Model file for the job. Use its own axes, mm. Face numbers are marked on the shaded views. A direction names the side the tool comes from. Coordinates: 2 decimals unless noted, no trailing zeros. Order: outer loops, then holes, each group sorted by start corner. A loop starts at its lowest first (then second) coordinate and runs counter-clockwise, first axis right, second up. Notation, with made-up numbers: M -7,73 L 4,73 A18 cw 4,104 Z; hole C 5,72.5 d11. An arc over 180 degrees is marked long. Return JSON: item names as keys, results as strings.
```python
from build123d import *

# Parameters (mm, degrees)
SKETCH_1_W      = 1800
SKETCH_1_H      = 870
EXTRUDE_1_DEPTH = 70
SKETCH_2_W      = 100
SKETCH_2_H      = 300
EXTRUDE_2_DEPTH = 150
SKETCH_3_W      = 300
SKETCH_3_H      = 300
EXTRUDE_3_DEPTH = 190
SKETCH_4_W      = 90
SKETCH_4_H      = 710
SKETCH_4_W_2    = 1460
SKETCH_4_H_2    = 90
EXTRUDE_4_DEPTH = 70
SKETCH_5_W      = 90
SKETCH_5_H      = 90
EXTRUDE_5_DEPTH = 600
EXTRUDE_6_REACH = 2071.251
SKETCH_6_W      = 90
SKETCH_6_H      = 90
EXTRUDE_7_REACH = 2013.641
SKETCH_7_W      = 650
SKETCH_7_H      = 90


with BuildPart() as part:
    # ｽｹｯﾁ1 → ﾎﾞｽ - 押し出し1 (new body)
    with BuildSketch(Plane(origin=(0, 0, 0), x_dir=(1, 0, 0), z_dir=(0, 1, 0))):
        with Locations((900, 435)):
            Rectangle(SKETCH_1_W, SKETCH_1_H)
    extrude(amount=EXTRUDE_1_DEPTH)

    # ｽｹｯﾁ2 → ﾎﾞｽ - 押し出し2 (add)
    with BuildSketch(Plane(origin=(0, 70, 0), x_dir=(1, 0, 0), z_dir=(0, 1, 0))):
        with Locations((350, 50)):
            Rectangle(SKETCH_2_W, SKETCH_2_H)
        with Locations((1450, 50)):
            Rectangle(SKETCH_2_W, SKETCH_2_H)
        with Locations((1450, 820)):
            Rectangle(SKETCH_2_W, SKETCH_2_H)
        with Locations((350, 820)):
            Rectangle(SKETCH_2_W, SKETCH_2_H)
    extrude(amount=EXTRUDE_2_DEPTH)

    # ｽｹｯﾁ3 → ﾎﾞｽ - 押し出し3 (add)
    with BuildSketch(Plane(origin=(0, 70, 0), x_dir=(1, 0, 0), z_dir=(0, 1, 0))):
        with Locations((900, 435)):
            Rectangle(SKETCH_3_W, SKETCH_3_H)
    extrude(amount=EXTRUDE_3_DEPTH)

    # ｽｹｯﾁ4 → ﾎﾞｽ - 押し出し4 (add)
    with BuildSketch(Plane(origin=(0, 0, 0), x_dir=(-1, 0, 0), z_dir=(0, -1, 0))):
        with Locations((-1675, 435)):
            Rectangle(SKETCH_4_W, SKETCH_4_H)
        with Locations((-900, 715)):
            Rectangle(SKETCH_4_W_2, SKETCH_4_H_2)
        with Locations((-900, 155)):
            Rectangle(SKETCH_4_W_2, SKETCH_4_H_2)
        with Locations((-125, 435)):
            Rectangle(SKETCH_4_W, SKETCH_4_H)
    extrude(amount=EXTRUDE_4_DEPTH)

    # ｽｹｯﾁ5 → ﾎﾞｽ - 押し出し5 (add)
    with BuildSketch(Plane(origin=(0, -70, 0), x_dir=(-1, 0, 0), z_dir=(0, -1, 0))):
        with Locations((-1675, 155)):
            Rectangle(SKETCH_5_W, SKETCH_5_H)
        with Locations((-1675, 715)):
            Rectangle(SKETCH_5_W, SKETCH_5_H)
        with Locations((-125, 155)):
            Rectangle(SKETCH_5_W, SKETCH_5_H)
        with Locations((-125, 715)):
            Rectangle(SKETCH_5_W, SKETCH_5_H)
    extrude(amount=EXTRUDE_5_DEPTH)

    # ｽｹｯﾁ6 → ﾎﾞｽ - 押し出し6 (add, up to next)
    with BuildSketch(Plane(origin=(0, 0, -200), x_dir=(-1, 0, 0), z_dir=(0, 0, -1)), mode=Mode.PRIVATE) as extrude_6_sk1:
        with Locations((-1675, -525)):
            Rectangle(SKETCH_6_W, SKETCH_6_H)
    extrude_6_tool1 = extrude(extrude_6_sk1.sketch, amount=EXTRUDE_6_REACH, mode=Mode.PRIVATE) - part.part
    # ｽｹｯﾁ6 → ﾎﾞｽ - 押し出し6 (add, up to next)
    with BuildSketch(Plane(origin=(0, 0, -200), x_dir=(-1, 0, 0), z_dir=(0, 0, -1)), mode=Mode.PRIVATE) as extrude_6_sk2:
        with Locations((-125, -525)):
            Rectangle(SKETCH_6_W, SKETCH_6_H)
    extrude_6_tool2 = extrude(extrude_6_sk2.sketch, amount=EXTRUDE_6_REACH, mode=Mode.PRIVATE) - part.part
    add(extrude_6_tool1.solids().sort_by_distance((1675, -525, -200))[0])
    add(extrude_6_tool2.solids().sort_by_distance((125, -525, -200))[0])

    # ｽｹｯﾁ7 → ﾎﾞｽ - 押し出し7 (add, up to next)
    with BuildSketch(Plane.ZY.offset(-1630), mode=Mode.PRIVATE) as extrude_7_sk1:
        with Locations((-435, -525)):
            Rectangle(SKETCH_7_W, SKETCH_7_H)
    extrude_7_tool1 = extrude(extrude_7_sk1.sketch, amount=EXTRUDE_7_REACH, mode=Mode.PRIVATE) - part.part
    add(extrude_7_tool1.solids().sort_by_distance((1630, -525, -435))[0])


solid = part.part
```
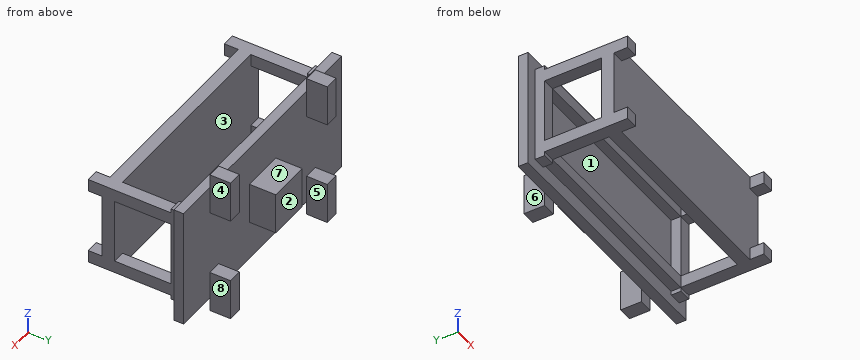
Item 1: Saw through at A-A (y = -328). Write the cut outline in (x, z).
Check result:
{"outline": "M 80,-760 L 170,-760 L 170,-670 L 80,-670 Z; M 80,-200 L 170,-200 L 170,-110 L 80,-110 Z; M 1630,-760 L 1720,-760 L 1720,-670 L 1630,-670 Z; M 1630,-200 L 1720,-200 L 1720,-110 L 1630,-110 Z"}
Item 2: Saw through at B-B (x = 768.5). Write the cut outline in (y, z).
Check result:
{"outline": "M -570,-760 L -480,-760 L -480,-110 L -570,-110 Z; M -70,-760 L 0,-760 L 0,-870 L 70,-870 L 70,-585 L 260,-585 L 260,-285 L 70,-285 L 70,0 L 0,0 L 0,-110 L -70,-110 L -70,-200 L 0,-200 L 0,-670 L -70,-670 Z"}
Item 3: Drop flat-ended pins along their axis: pin 1 Ø24 at (y, z) = (-44.5, -100) entering from -X; pin 2 Ø24 at (y, z) = (-44.5, -94.5) entering from +X; pin 3 Ø1.5 at (x, z) = (285, -122.5) entering from +Y; pin 4 Ø1.5 at (y, z) = (-206.5, -667.5) entering from -X. Give the stop position or say it passes through.
Check result:
{"pin 1": "stops at x = 80", "pin 2": "stops at x = 1720", "pin 3": "stops at y = 70", "pin 4": "passes through"}
Item 4: Pull direction Y, two halves, no side cores. Call the marked faces 1, 2, 3 and 4: +Y half, -Y half, draft (parallel to the pull), parting line (faces both ways), or undercut.
Check result:
{"face 1": "undercut", "face 2": "+Y half", "face 3": "undercut", "face 4": "draft"}
Item 5: Saw through at D-D (x = 1668). Write the cut outline in (y, z), and give its area (3 significant figures).
Check result:
{"outline": "M -670,-760 L -70,-760 L -70,-790 L 0,-790 L 0,-870 L 70,-870 L 70,0 L 0,0 L 0,-80 L -70,-80 L -70,-110 L -670,-110 L -670,-200 L -570,-200 L -570,-670 L -670,-670 Z; hole M -480,-670 L -70,-670 L -70,-200 L -480,-200 Z", "area": "261,000 mm2"}
Item 6: 3-axis set-ups, long thin cutter, end or side, ignore diameter. For the marked faces 5, 6, 7 and 8: which of +Z, -Z, +X, -X, +Y, -Y reach the whole face in a straight line?
Check result:
{"face 5": "+Z, -Z, +Y", "face 6": "+Z, -Z, -X, +Y", "face 7": "+Z, +X, -X, +Y", "face 8": "+Z, -Z, +X, +Y"}
Item 7: Wall check: line 1 (Z direction, x = 1654, y = -618.5); line 2 (Y direction, x = 516.5, z = -217); line 3 (X direction, y = -237, z = -679). Give the ranges that are in metal, low to high.
Check result:
{"line 1": "z = -760 to -670, -200 to -110", "line 2": "y = -570 to -480, 0 to 70", "line 3": "x = 80 to 170, 1630 to 1720"}
Item 8: Saw through at C-C (z = -502). Write the cut outline in (x, y).
Check result:
{"outline": "M 0,0 L 80,0 L 80,-70 L 170,-70 L 170,0 L 1630,0 L 1630,-70 L 1720,-70 L 1720,0 L 1800,0 L 1800,70 L 1050,70 L 1050,260 L 750,260 L 750,70 L 0,70 Z; M 80,-570 L 1720,-570 L 1720,-480 L 80,-480 Z"}
